Part model, mm, in its own coordinate system. Face numbers are marked on the shaded views. A direction names the side the tool comes from. Give positions to 0.01 mm unless a question says otherwise; leave off trailing zeros. Order: outer loops, then holes, each group sorted by start corner. A loop starts at its lowest first (then second) coordinate and runs counter-clockwise, first axis right, second up. Notation, with made-up numbers: (58.5, 60) - (75.5, 60) arc R5 ccw to (75.5, 69) - close; hole circle Ø3 at (42.25, 2.25). An arc over 180 degrees is marked (long way). Use a Markdown table: item, result. Add a question column.
from build123d import *

# Parameters (mm, degrees)
F0_W           = 5
F0_H           = 65
F0_W_2         = 240
F1_DEPTH       = 5
F2_W           = 5
F2_H           = 65
F3_DEPTH       = 65
F4_R           = 6.477
F5_DEPTH       = 250.001
F6_R           = 6.477
F7_DEPTH       = 25.4
F8_W           = 90
F8_H           = 35
F9_DEPTH       = 25.4
F10_W          = 35
F10_H          = 18.523
F11_DEPTH      = 245.001
F11_DEPTH_BACK = 25.4
F12_R          = 1.5
F13_DEPTH      = 25.4
F12_W          = 25
F12_H          = 7
F12_R_2        = 1
F14_DEPTH      = 5
F15_R          = 13.335
F15_R_2        = 6.477
F16_DEPTH      = 3
F17_R          = 1.143
F18_DEPTH      = 2.001
F19_R          = 1.143
F20_DEPTH      = 250.001


# Not quite as in the source:
# - a feature names something its author has since deleted; it is built from what else it names


with BuildPart() as f1:
    # F0 (on Top) → F1 (new body)
    with BuildSketch(Plane.XY):
        with Locations((-114.2006202787, -15.5218991437)):
            Rectangle(F0_W, F0_H)
        with Locations((130.7993797213, -15.5218991437)):
            Rectangle(F0_W, F0_H)
        with Locations((8.2993797213, -15.5218991437)):
            Rectangle(F0_W_2, F0_H)
    extrude(amount=F1_DEPTH)

    # F2 (on face) → F3 (join)
    with BuildSketch(Plane(origin=(0, 0, 0), x_dir=(1, 0, 0), z_dir=(0, 0, -1))):
        with Locations((-114.2006202787, 15.5218991437)):
            Rectangle(F2_W, F2_H)
        with Locations((130.7993797213, 15.5218991437)):
            Rectangle(F2_W, F2_H)
    extrude(amount=F3_DEPTH)

    # F4 (on face) → F5 (cut, through all)
    with BuildSketch(Plane.YZ.offset(133.2993797213)):
        with Locations((-15.5218991437, -50)):
            Circle(F4_R)
    extrude(amount=-F5_DEPTH, mode=Mode.SUBTRACT)

    # F6 (on face) → F7 (cut)
    with BuildSketch(Plane(origin=(0, 0, 0), x_dir=(1, 0, 0), z_dir=(0, 0, -1))):
        with Locations((8.2993797213, 15.5218991437)):
            Circle(F6_R)
    extrude(amount=-F7_DEPTH, mode=Mode.SUBTRACT)

    # F8 (on face) → F9 (cut)
    with BuildSketch(Plane(origin=(0, 0, 0), x_dir=(1, 0, 0), z_dir=(0, 0, -1))):
        with Locations((-56.7006202787, 15.5218991437)):
            Rectangle(F8_W, F8_H)
        with Locations((73.2993797213, 15.5218991437)):
            Rectangle(F8_W, F8_H)
    extrude(amount=-F9_DEPTH, mode=Mode.SUBTRACT)

    # F10 (on face) → F11 (cut, two sides)
    with BuildSketch(Plane.YZ.offset(-111.7006202787)) as f11_sk:
        with Locations((-15.5218991437, -19.2615)):
            Rectangle(F10_W, F10_H)
    extrude(amount=F11_DEPTH, mode=Mode.SUBTRACT)
    extrude(f11_sk.sketch, amount=-F11_DEPTH_BACK, mode=Mode.SUBTRACT)

    # F12 (on face) → F13 (cut)
    with BuildSketch(Plane.YZ.offset(133.2993797213)):
        with Locations((-23.0218991437, 0)):
            Circle(F12_R)
        with Locations((-8.0218991437, 0)):
            Circle(F12_R)
    extrude(amount=-F13_DEPTH, mode=Mode.SUBTRACT)

    # F12 (on face) → F14 (join, through all)
    with BuildSketch(Plane.YZ.offset(133.2993797213)):
        with Locations((-15.5218991437, -68.5)):
            Rectangle(F12_W, F12_H)
        with Locations((-23.0218991437, -67)):
            Circle(F12_R_2, mode=Mode.SUBTRACT)
        with Locations((-8.0218991437, -67)):
            Circle(F12_R_2, mode=Mode.SUBTRACT)
    extrude(amount=-F14_DEPTH)

    # F15 (on face) → F16 (cut)
    with BuildSketch(Plane(origin=(0, 0, 0), x_dir=(1, 0, 0), z_dir=(0, 0, -1))):
        with Locations((8.2993797213, 15.5218991437)):
            Circle(F15_R)
        with Locations((8.2993797213, 15.5218991437)):
            Circle(F15_R_2, mode=Mode.SUBTRACT)
    extrude(amount=-F16_DEPTH, mode=Mode.SUBTRACT)

    # F17 (on face) → F18 (cut, through all)
    with BuildSketch(Plane(origin=(0, 0, 3), x_dir=(1, 0, 0), z_dir=(0, 0, -1))):
        with Locations((14.6909433031, 22.9230312179)):
            Circle(F17_R)
        with Locations((18.0783797213, 15.5218991437)):
            Circle(F17_R)
        with Locations((15.2324973507, 8.6286974185)):
            Circle(F17_R)
        with Locations((8.8073272824, 5.7887949694)):
            Circle(F17_R)
        with Locations((1.9078161395, 8.1207670695)):
            Circle(F17_R)
        with Locations((-1.4796202787, 15.5218991437)):
            Circle(F17_R)
        with Locations((1.3662620919, 22.415100869)):
            Circle(F17_R)
        with Locations((7.7914321602, 25.2550033181)):
            Circle(F17_R)
    extrude(amount=-F18_DEPTH, mode=Mode.SUBTRACT)

    # F19 (on face) → F20 (cut, through all)
    with BuildSketch(Plane(origin=(-116.7006202787, 0, 0), x_dir=(0, -1, 0), z_dir=(-1, 0, 0))):
        with Locations((15.765312519, -40.2836638916)):
            Circle(F19_R)
        with Locations((25.1764905212, -49.2415353535)):
            Circle(F19_R)
        with Locations((23.1101417116, -56.0547046433)):
            Circle(F19_R)
        with Locations((15.2784857684, -59.7163361084)):
            Circle(F19_R)
        with Locations((8.2459797528, -56.5320689682)):
            Circle(F19_R)
        with Locations((5.8673077662, -50.7584646465)):
            Circle(F19_R)
        with Locations((7.9336565759, -43.9452953567)):
            Circle(F19_R)
        with Locations((22.7978185346, -43.4679310318)):
            Circle(F19_R)
    extrude(amount=-F20_DEPTH, mode=Mode.SUBTRACT)


solid = f1.part
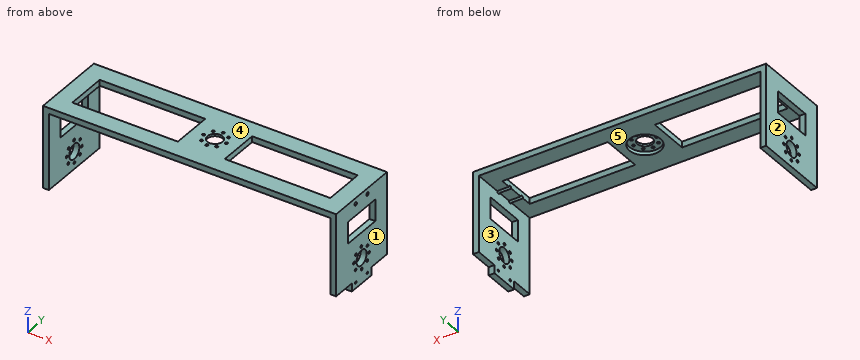
1. Mould opens along X. For the marked faces 1, 2 and 3 say: released by +X, released by -X, zero draft, split by the parting line, or undercut.
2. Cut at A-A (x = -91). Write the cut outline in (y, z), plus the area to 3 significant figures.
3. Pin check, flat tip, straight feed: P1, Ø1.5, axis at x = -114, y = -15.5, coming from the -Z side. Stop position of the tip, or through.
4. Drill centre lines: probe 1 along X at (y, z) = (-24.5, -62); probe 2 along Z at (x, y) = (-62, -35). Where is each one in solid material? Low to high. Write a range as [from, to].
5. Cut at B-B (y = -38). Write the cut outline in (x, z).
6. Tool access for the marked faces 4 and 5: list every direction of +Z, -Z, +X, -X, +Y, -Y with a clear straight run to the whole face (end or side of a thin tool).
7. Cut at C-C (x = -7.5). Write the cut outline in (y, z), plus the area to 3 significant figures.
Responses:
| question | item | result |
|---|---|---|
| 1 | face 1 | released by +X |
| 1 | face 2 | released by -X |
| 1 | face 3 | undercut |
| 2 | outline | (-48.02, 0) - (-33.02, 0) - (-33.02, 5) - (-48.02, 5) - close; (1.98, 0) - (16.98, 0) - (16.98, 5) - (1.98, 5) - close |
| 2 | area | 150 mm² |
| 3 | P1 | stops at z = -65 |
| 4 | probe 1 | x = [-116.7, -111.7], [128.3, 133.3] |
| 4 | probe 2 | z = [0, 5] |
| 5 | outline | (-116.7, -65) - (-111.7, -65) - (-111.7, 0) - (128.3, 0) - (128.3, -65) - (133.3, -65) - (133.3, 5) - (-116.7, 5) - close |
| 6 | face 4 | +Z, +X, -X, +Y, -Y |
| 6 | face 5 | -Z, +Y, -Y |
| 7 | outline | (-48.02, 0) - (16.98, 0) - (16.98, 5) - (-48.02, 5) - close |
| 7 | area | 325 mm² |
